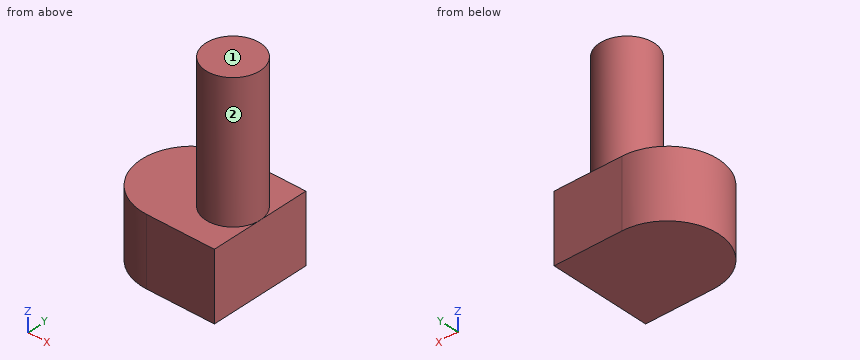
```python
from build123d import *

# Parameters (mm, degrees)
F2_DEPTH = 6.35
F1_R     = 2.54
F3_DEPTH = 19.05


with BuildPart() as f2:
    # F0 (on Top) → F2 (new body)
    with BuildSketch(Plane.XY):
        with BuildLine():
            Line((6.35, 4.7625), (0, 4.7625))
            ThreePointArc((0, 4.7625), (-4.7625, 0), (0, -4.7625))
            Line((0, -4.7625), (6.35, -4.7625))
            Line((6.35, -4.7625), (6.35, 4.7625))
        make_face()
    extrude(amount=F2_DEPTH)

    # F1 (on Top) → F3 (join)
    with BuildSketch(Plane.XY):
        with Locations((3.81, 0)):
            Circle(F1_R)
    extrude(amount=F3_DEPTH)


solid = f2.part
```
Geometry: final body of the model. Coordinates: model frame, mm. Face numbers are marked on the shaded views. A direction names the side the tool comes from. Coordinates: 2 decimals unless noted, no trailing zeros. Order: outer loops, then holes, each group sorted by start corner. A loop starts at its lowest first (then second) coordinate and runs counter-clockwise, first axis right, second up. Notation, with made-up numbers: M 80.5,-35 L 106.5,-35 A9 ccw 106.5,-18 Z; hole C 71.25,39.5 d6. An arc over 180 degrees is marked long. Answer in a Markdown table with one row per item. Add a question column.
Q1. Section query D-D on y = 3.5. Return the cut outline in (x, z).
Q2. Section query B-B on y = -0.5. Return the cut outline in (x, z).
Q3. Contact query for flat-ended pins moving along their axis: P1, Ø3, axis at y = -3, z = 10, coming from the -X side; P2, Ø2, axis at x = -3.5, y = -3, coming from the -Z side; P3, Ø1, axis at x = -2.5, y = 2, coming from the +Z side; P4, Ø5, axis at x = 4, z = 14, coming from the -Y side. Output: stop coordinate, or through.
Q4. Section query A-A on x = 3.81. Return the cut outline in (y, z).
Q5. Line query: L1, parallel to Z at x = -3.75, y = -0.5; L2, parallel to Y at x = 4.5, z = 6.5; L3, parallel to X at y = 0.25, z = 16. Output: solid intervals per line, ascending.
Q6. Reachability of the marked faces 1 and 2 from +Z, -Z, +X, -X, +Y, -Y: full face, straight path, thin tool, end or side. Return the list, or none.
Completed:
| question | item | result |
|---|---|---|
| 1 | outline | M -3.23,0 L 6.35,0 L 6.35,6.35 L -3.23,6.35 Z |
| 2 | outline | M -4.74,0 L 6.35,0 L 6.35,6.35 L 6.3,6.35 L 6.3,19.05 L 1.32,19.05 L 1.32,6.35 L -4.74,6.35 Z |
| 3 | P1 | stops at x = 1.76 |
| 3 | P2 | stops at z = 0 |
| 3 | P3 | stops at z = 6.35 |
| 3 | P4 | stops at y = -2.54 |
| 4 | outline | M -4.76,0 L 4.76,0 L 4.76,6.35 L 2.54,6.35 L 2.54,19.05 L -2.54,19.05 L -2.54,6.35 L -4.76,6.35 Z |
| 5 | L1 | z = 0 to 6.35 |
| 5 | L2 | y = -2.44 to 2.44 |
| 5 | L3 | x = 1.28 to 6.34 |
| 6 | face 1 | +Z, +X, -X, +Y, -Y |
| 6 | face 2 | +Z |
